from build123d import *

# Parameters (mm, degrees)
IZIM1_W                     = 28
IZIM1_H                     = 28
Y_KSEKLIK_EKSTR_ZYON1_DEPTH = 585
IZIM2_R                     = 6
KES_EKSTR_ZYON1_DEPTH       = 60
SKETCH1_R                   = 3
CUT_EXTRUDE1_DEPTH          = 10
SKETCH2_R                   = 3
CUT_EXTRUDE2_DEPTH          = 586.837008049
SKETCH3_R                   = 4.25
CUT_EXTRUDE3_DEPTH          = 6
SKETCH4_W                   = 79.561179617
SKETCH4_H                   = 84.218096563
SKETCH4_W_2                 = 144.712868034
SKETCH4_H_2                 = 206.469543182
CUT_EXTRUDE4_DEPTH          = 0.3


with BuildPart() as part:
    # Çizim1 → Yükseklik-Ekstrüzyon1 (new body)
    with BuildSketch(Plane.XY):
        Rectangle(IZIM1_W, IZIM1_H)
    extrude(amount=Y_KSEKLIK_EKSTR_ZYON1_DEPTH)

    # Çizim2 → Kes-Ekstrüzyon1 (cut)
    with BuildSketch(Plane.XY.offset(585)):
        Circle(IZIM2_R)
    extrude(amount=-KES_EKSTR_ZYON1_DEPTH, mode=Mode.SUBTRACT)

    # Sketch1 → Cut-Extrude1 (cut)
    with BuildSketch(Plane(origin=(0, 0, 0), x_dir=(-1, 0, 0), z_dir=(0, 0, -1))):
        with Locations((-7, -7)):
            Circle(SKETCH1_R)
        with Locations((7, 7)):
            Circle(SKETCH1_R)
    extrude(amount=-CUT_EXTRUDE1_DEPTH, mode=Mode.SUBTRACT)

    # Sketch2 → Cut-Extrude2 (cut, through all)
    with BuildSketch(Plane.ZY.offset(14)):
        with Locations((485, 0)):
            Circle(SKETCH2_R)
    extrude(amount=-CUT_EXTRUDE2_DEPTH, mode=Mode.SUBTRACT)

    # Sketch3 → Cut-Extrude3 (cut)
    with BuildSketch(Plane.ZY.offset(14)):
        with Locations((485, 0)):
            Circle(SKETCH3_R)
    extrude(amount=-CUT_EXTRUDE3_DEPTH, mode=Mode.SUBTRACT)

    # Sketch4 → Cut-Extrude4 (cut)
    with BuildSketch(Plane.ZY.offset(14)):
        with Locations((591.780589809, 6.31374468)):
            Rectangle(SKETCH4_W, SKETCH4_H)
        with Locations((-12.856434017, 14.64786351)):
            Rectangle(SKETCH4_W_2, SKETCH4_H_2)
    extrude(amount=-CUT_EXTRUDE4_DEPTH, mode=Mode.SUBTRACT)


solid = part.part
Design review of the part built by this model. Coordinates are the model's own, in mm. Round coordinates to 2 decimals unless told otherwise and drop trailing zeros.
1) For L1, parallel to Z at x = -12.25, y = 3; L2, parallel to Y at x = -10.15, z = 485; L3, parallel to Y at x = -1.75, z = 485, list the stretches that pass through material, from the lowest coordinate up.
The answers:
L1: z = 0 to 481.99, 488.01 to 585
L2: y = -14 to -4.25, 4.25 to 14
L3: y = -14 to -3, 3 to 14
2) Draft analysis for pull direction X (two halves, no side actions). For faces 1 (the flat face through (14, 0, 288)), 2 (the flat face through (0, -14, 288)), 3 (the cylindrical face through (-6, 0, 555)), 4 (the flat face through (-14, 0, 302)), state which applies: released by +X, released by -X, zero draft, split by the parting line, or undercut.
The answers:
face 1: released by +X
face 2: zero draft
face 3: undercut
face 4: released by -X
3) Clearance check with flat-ended pins moving along their axes: pin 1 Ø1.5 at (x, y) = (-4, -3) entering from +Z; pin 2 Ø3.5 at (x, y) = (-7, 7) entering from -Z. State where each tip first meets the part, or that it passes through.
The answers:
pin 1: stops at z = 525
pin 2: stops at z = 10
